from build123d import *

# Parameters (mm, degrees)
SKETCH1_W           = 139
SKETCH1_H           = 139
BOSS_EXTRUDE1_DEPTH = 6.35
FILLET1_R           = 10.56
SKETCH2_W           = 93
SKETCH2_H           = 93
SLOTCUT_DEPTH       = 100.104944377


with BuildPart() as part:
    # Sketch1 → Boss-Extrude1 (new, symmetric)
    with BuildSketch(Plane(origin=(0, 0, 0), x_dir=(1, 0, 0), z_dir=(0, 1, 0))):
        Rectangle(SKETCH1_W, SKETCH1_H)
    extrude(amount=BOSS_EXTRUDE1_DEPTH, both=True)

    # Fillet1
    fillet1_edges = [part.edges().sort_by_distance(p)[0] for p in [
        (69.5, 0, 69.5),
        (-69.5, 0, 69.5),
        (-69.5, 0, -69.5),
        (69.5, 0, -69.5),
    ]]
    fillet(fillet1_edges, radius=FILLET1_R)

    # Sketch2 → SlotCut (cut, through all)
    with BuildSketch(Plane(origin=(0, 6.35, 0), x_dir=(1, 0, 0), z_dir=(0, 1, 0))):
        Rectangle(SKETCH2_W, SKETCH2_H)
    extrude(amount=-SLOTCUT_DEPTH, mode=Mode.SUBTRACT)


solid = part.part
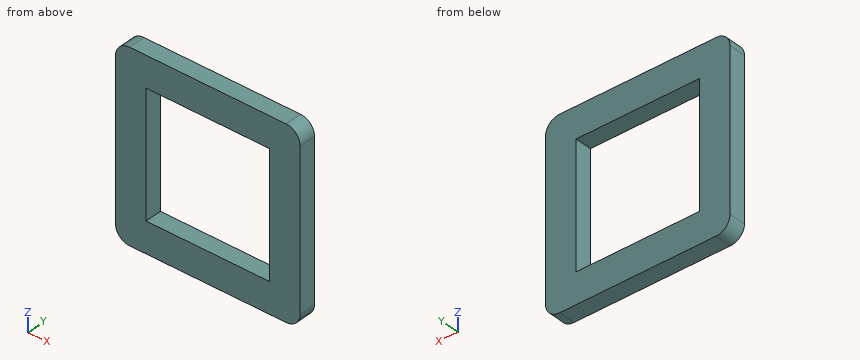
Can you work these out from the model? Positions are in its coordinate system, mm. Coordinates: 2 decimals unless noted, no trailing zeros. Order: outer loops, then holes, each group sorted by start corner. A loop starts at its lowest first (then second) coordinate and runs counter-clockwise, first axis right, second up. Notation, with made-up numbers: M 55,0 L 113,0 A22 cw 113,12 Z; hole C 23.5,-30 d10. An arc over 180 degrees is marked long. Answer as CSV lines item,"result".
(1) Suppose I cut it at A-A on z = -33. Please give me the cut outline in (x, y), plus the area to 3 significant figures.
Geometry check:
outline,"M -69.5,-6.35 L -46.5,-6.35 L -46.5,6.35 L -69.5,6.35 Z; M 46.5,-6.35 L 69.5,-6.35 L 69.5,6.35 L 46.5,6.35 Z"
area,"584 mm^2"
(2) Suppose I cut it at B-B on y = -3.25. Please give me the cut outline in (x, z).
Geometry check:
outline,"M -69.5,-58.94 A10.56 ccw -58.94,-69.5 L 58.94,-69.5 A10.56 ccw 69.5,-58.94 L 69.5,58.94 A10.56 ccw 58.94,69.5 L -58.94,69.5 A10.56 ccw -69.5,58.94 Z; hole M -46.5,-46.5 L 46.5,-46.5 L 46.5,46.5 L -46.5,46.5 Z"
(3) Suppose I cut it at C-C on x = -26. Please give me the cut outline in (y, z), plus the area to 3 significant figures.
Geometry check:
outline,"M -6.35,-69.5 L 6.35,-69.5 L 6.35,-46.5 L -6.35,-46.5 Z; M -6.35,46.5 L 6.35,46.5 L 6.35,69.5 L -6.35,69.5 Z"
area,"584 mm^2"
(4) Please list where these lines run through material, in increasing order: L1, parallel to X at y = -4.5, z = 0.5; L2, parallel to Z at x = 60, y = -5.5.
Geometry check:
L1,"-69.5 to -46.5, 46.5 to 69.5"
L2,"-69.45 to 69.45"
